The listing builds one solid part. Answer for the finished solid, in the listing's coordinates (mm). Face numbers are marked on the shaded views. A direction names the side the tool comes from. Give positions to 0.01 mm unless a question says otherwise; leave off trailing zeros. Write each loop counter-clockwise with the first axis right and the second up, starting at its lowest first coordinate (ties: lowest second). Pieces come first, ordered by that corner, then holes. Notation, with made-up numbers: M 1.25,-15 L 52.25,-15 A9 cw 52.25,-4 Z; hole C -0.5,74 d6. An arc over 180 degrees is marked long. Return JSON: item names as keys, results as strings.
from build123d import *

# Parameters (mm, degrees)
HOLE1_D     = 13.5128
HOLE1_DEPTH = 18.5928
HOLE1_TIP   = 3.900809359
SKETCH5_W   = 6.35
SKETCH5_H   = 12.3063


with BuildPart() as part:
    # Sketch1 → Revolve1 (revolve)
    with BuildSketch(Plane.XY, mode=Mode.PRIVATE) as revolve1_sk:
        Polygon((0, 0), (0, 18.43405), (0.762, 19.19605), (4.318, 19.19605), (5.334, 18.18005), (6.35, 18.18005), (6.35, 19.76755), (21.463, 19.76755), (22.225, 19.00555), (22.225, 0), align=None)
    revolve(revolve1_sk.sketch.rotate(Axis((22.225, 0, 0), (-1, 0, 0)), 270), axis=Axis((22.225, 0, 0), (-1, 0, 0)))

    # Hole1
    with Locations(Plane.ZY):
        with Locations((0, 0)):
            Hole(HOLE1_D / 2, depth=HOLE1_DEPTH)
            with Locations((0, 0, -(HOLE1_DEPTH + HOLE1_TIP / 2))):  # 120° drill point
                Cone(0, HOLE1_D / 2, HOLE1_TIP, mode=Mode.SUBTRACT)

    # Sketch4 → Cut-Revolve1 (revolve, cut)
    with BuildSketch(Plane(origin=(0, 0, 0), x_dir=(1, 0, 0), z_dir=(0, 1, 0)), mode=Mode.PRIVATE) as cut_revolve1_sk:
        Polygon((14.2748, 0), (18.86262618, 0), (18.86262618, -11.706901754), (19.094451116, -19.132537191), (19.729463925, -19.76755), (14.2748, -19.76755), align=None)
    revolve(cut_revolve1_sk.sketch.rotate(Axis((14.2748, 0, 19.76755), (0, 0, -1)), 180), axis=Axis((14.2748, 0, 19.76755), (0, 0, -1)), mode=Mode.SUBTRACT)

    # Sketch5 → Cut-Revolve2 (revolve, cut)
    with BuildSketch(Plane.XY, mode=Mode.PRIVATE) as cut_revolve2_sk:
        with Locations((3.175, 6.15315)):
            Rectangle(SKETCH5_W, SKETCH5_H)
    revolve(cut_revolve2_sk.sketch.rotate(Axis((6.35, 0, 0), (-1, 0, 0)), 270), axis=Axis((6.35, 0, 0), (-1, 0, 0)), mode=Mode.SUBTRACT)

    # Sketch6 → Revolve2 (revolve)
    with BuildSketch(Plane.XY, mode=Mode.PRIVATE) as revolve2_sk:
        with BuildLine():
            Line((5.267509175, 19.683381804), (6.216617928, 18.734273051))
            ThreePointArc((6.216617928, 18.734273051), (6.253815367, 18.64447049), (6.216617928, 18.554667928))
            Line((6.216617928, 18.554667928), (5.842, 18.18005))
            Line((5.842, 18.18005), (5.334, 18.18005))
            Line((5.334, 18.18005), (5.334, 17.92605))
            Line((5.334, 17.92605), (6.35, 17.92605))
            Line((6.35, 17.92605), (6.35, 18.888259175))
            Line((6.35, 18.888259175), (5.470709175, 19.76755))
            Line((5.470709175, 19.76755), (5.267509175, 19.76755))
            Line((5.267509175, 19.76755), (5.267509175, 19.683381804))
        make_face()
    revolve(revolve2_sk.sketch.rotate(Axis((6.35, 0, 0), (-1, 0, 0)), 270), axis=Axis((6.35, 0, 0), (-1, 0, 0)))


solid = part.part
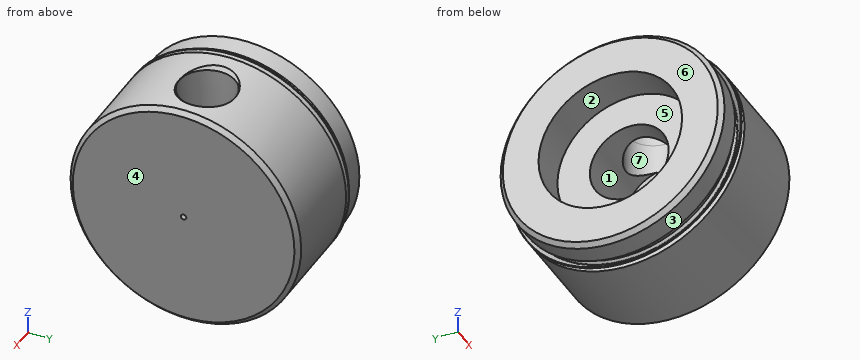
Item 1: Find the intervals of material crossed by line 1 (X direction, y = 0, z = 9.25) (3 decimals); line 2 (Y direction, x = 13.25, z = 0); line 3 (X direction, y = -8, z = 0) (3 decimals), in increasing order.
Geometry results:
{"line 1": "x = 6.35 to 9.687, 18.863 to 22.225", "line 2": "y = -19.77 to -6.76, 6.76 to 19.77", "line 3": "x = 6.35 to 22.225"}
Item 2: Determine the mould class of the marked faces 1, 2, 3 and 4 for opening direction Z: +Z half, -Z half, draft (parallel to the pull), parting line (faces both ways), or undercut.
Geometry results:
{"face 1": "undercut", "face 2": "undercut", "face 3": "parting line", "face 4": "draft"}
Item 3: Given pin 1 Ø12 at (y, z) = (6.5, 6.5) entering from -X; pin 2 Ø12 at (x, y) = (4, 15.5) entering from +Z; pin 3 Ø12.5 at (y, z) = (4, -2) entering from -X; pin 4 Ø12 at (y, z) = (0, 0) entering from -X, each flat-ended and moving along its own axis, determine where each tip first touches the part or whether it passes through.
Geometry results:
{"pin 1": "stops at x = 0", "pin 2": "stops at z = 17.26", "pin 3": "stops at x = 6.35", "pin 4": "stops at x = 19.03"}
Item 4: A cutting plane is placed at C-C, the plane x = 20.75. Write down the section's boundary in (y, z), plus the area to 3 significant figures.
Geometry results:
{"outline": "C 0,0 d39.54; hole C 0,0 d6.04", "area": "1,200 mm2"}
Item 5: A cutting plane is placed at B-B, the plane y = 0. Count the separate pieces of the cut face and the enclosed holes in it, plus the area to 3 significant figures.
Geometry results:
{"separate pieces": "3", "enclosed holes": "0", "area": "398 mm2"}
Item 6: A cutting plane is placed at A-A, the plane x = 3.75. Write down the section's boundary in (y, z), plus the area to 3 significant figures.
Geometry results:
{"outline": "C 0,0 d38.39; hole C 0,0 d24.61", "area": "682 mm2"}
Item 7: Which of the six approach directions +Z, -Z, +X, -X, +Y, -Y give full straight-line access (tool end or side, diameter ignored) to the marked faces 5, 6 and 7?
Geometry results:
{"face 5": "-X", "face 6": "+Z, -Z, -X, +Y, -Y", "face 7": "+Z"}
